CAD build for the part. Positions are in the model's coordinates, mm. Face numbers are marked on the shaded views. A direction names the side the tool comes from. Give positions to 0.01 mm unless a question says otherwise; leave off trailing zeros. Loops run counter-clockwise (first coordinate to the right, second up) from the corner with the lowest first, then second, coordinate; pieces in that order, holes last. Notation, with made-up numbers: (60, 83) - (82, 83) arc R34 ccw to (82, 115) - close; hole circle Ø5 at (-28.75, 88.25). An arc over 180 degrees is marked (long way). Return JSON: item names as keys, results as strings.
from build123d import *

# Parameters (mm, degrees)
SKETCH1_W           = 80
SKETCH1_H           = 160
BOSS_EXTRUDE1_DEPTH = 80
SHELL1_T            = -3
SKETCH2_W           = 40
SKETCH2_H           = 30
CUT_EXTRUDE1_DEPTH  = 70
SKETCH3_W           = 20
SKETCH3_H           = 15
CUT_EXTRUDE2_DEPTH  = 70
SKETCH4_W           = 70
SKETCH4_H           = 15
CUT_EXTRUDE3_DEPTH  = 70
SKETCH5_W           = 20
SKETCH5_H           = 10
SKETCH5_R           = 2
BOSS_EXTRUDE2_DEPTH = 3
SKETCH6_R           = 2
CUT_EXTRUDE4_DEPTH  = 3


with BuildPart() as part:
    # Sketch1 → Boss-Extrude1 (new body)
    with BuildSketch(Plane.XY):
        Rectangle(SKETCH1_W, SKETCH1_H)
    extrude(amount=BOSS_EXTRUDE1_DEPTH)

    # Shell1
    shell1_openings = [part.faces().sort_by_distance(p)[0] for p in [
        (0, 0, 0),
    ]]
    offset(amount=SHELL1_T, openings=shell1_openings, kind=Kind.INTERSECTION)

    # Sketch2 → Cut-Extrude1 (cut)
    with BuildSketch(Plane(origin=(0, 80, 0), x_dir=(1, 0, 0), z_dir=(0, 1, 0))):
        with Locations((0, -50)):
            Rectangle(SKETCH2_W, SKETCH2_H)
    extrude(amount=-CUT_EXTRUDE1_DEPTH, mode=Mode.SUBTRACT)

    # Sketch3 → Cut-Extrude2 (cut)
    with BuildSketch(Plane(origin=(0, 80, 0), x_dir=(1, 0, 0), z_dir=(0, 1, 0))):
        with Locations((0, -7.5)):
            Rectangle(SKETCH3_W, SKETCH3_H)
    extrude(amount=-CUT_EXTRUDE2_DEPTH, mode=Mode.SUBTRACT)

    # Sketch4 → Cut-Extrude3 (cut)
    with BuildSketch(Plane(origin=(0, -80, 0), x_dir=(-1, 0, 0), z_dir=(0, -1, 0))):
        with Locations((0, -7.5)):
            Rectangle(SKETCH4_W, SKETCH4_H)
    extrude(amount=-CUT_EXTRUDE3_DEPTH, mode=Mode.SUBTRACT)

    # Sketch5 → Boss-Extrude2 (add)
    # profile 1 of 2: a face of its own
    with BuildSketch(Plane(origin=(0, 0, 0), x_dir=(-1, 0, 0), z_dir=(0, 0, -1))):
        with Locations((50, 60)):
            Rectangle(SKETCH5_W, SKETCH5_H)
        with Locations((55, 60)):
            Circle(SKETCH5_R, mode=Mode.SUBTRACT)
    # profile 2 of 2: a face of its own
    with BuildSketch(Plane(origin=(0, 0, 0), x_dir=(-1, 0, 0), z_dir=(0, 0, -1))):
        with Locations((50, -70)):
            Rectangle(SKETCH5_W, SKETCH5_H)
        with Locations((55, -70)):
            Circle(SKETCH5_R, mode=Mode.SUBTRACT)
    boss_extrude2 = extrude(amount=-BOSS_EXTRUDE2_DEPTH)

    # Mirror1: Boss-Extrude2 across plane
    add(boss_extrude2.mirror(Plane(origin=(0, 0, 0), x_dir=(0, 0, 1), z_dir=(1, 0, 0))))

    # Sketch6 → Cut-Extrude4 (cut)
    with BuildSketch(Plane(origin=(0, 80, 0), x_dir=(1, 0, 0), z_dir=(0, 1, 0))):
        with Locations(Location((-27.5, -28, 0), (0, 0, 270))):
            Circle(SKETCH6_R)
        with Locations(Location((27.5, -28, 0), (0, 0, 270))):
            Circle(SKETCH6_R)
        with Locations(Location((27.5, -73, 0), (0, 0, 270))):
            Circle(SKETCH6_R)
        with Locations(Location((-27.5, -73, 0), (0, 0, 270))):
            Circle(SKETCH6_R)
    extrude(amount=-CUT_EXTRUDE4_DEPTH, mode=Mode.SUBTRACT)


solid = part.part
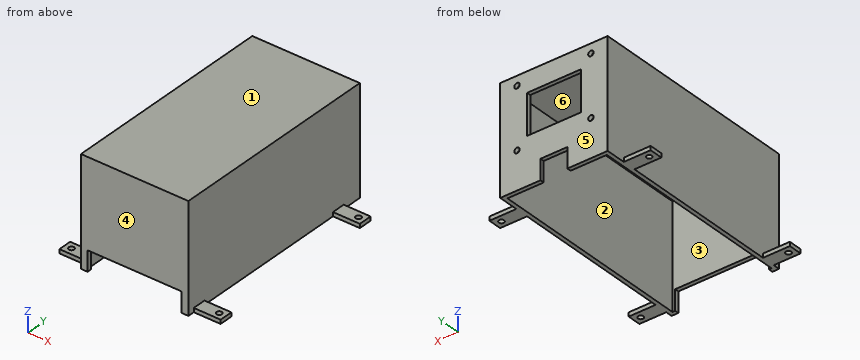
1. Cut at A-A, the plane z = 73. Write the cut outline in (x, y).
Values follow:
{"outline": "(-40, -80) - (40, -80) - (40, 80) - (29.5, 80) - (29.5, 77) - (37, 77) - (37, -77) - (-37, -77) - (-37, 77) - (-29.5, 77) - (-29.5, 80) - (-40, 80) - close; (-25.5, 77) - (25.5, 77) - (25.5, 80) - (-25.5, 80) - close"}
2. Pull direction Y, two halves, no side cores. Call the marked faces 3, 4, 5 and 6: +Y half, -Y half, draft (parallel to the pull), parting line (faces both ways), or undercut.
Values follow:
{"face 3": "undercut", "face 4": "-Y half", "face 5": "+Y half", "face 6": "undercut"}
3. Cut at B-B, the plane y = -70. Write the cut outline in (x, z).
Values follow:
{"outline": "(-60, 0) - (-57, 0) - (-57, 3) - (-60, 3) - close; (-53, 0) - (-37, 0) - (-37, 77) - (37, 77) - (37, 0) - (53, 0) - (53, 3) - (40, 3) - (40, 80) - (-40, 80) - (-40, 3) - (-53, 3) - close; (57, 0) - (60, 0) - (60, 3) - (57, 3) - close"}
4. Cut at D-D, the plane x = 42. Write the cut outline in (y, z).
Values follow:
{"outline": "(-75, 0) - (-65, 0) - (-65, 3) - (-75, 3) - close; (55, 0) - (65, 0) - (65, 3) - (55, 3) - close"}
5. Drill centre lines: probe 1 along X at (y, z) = (77.65, 28); probe 2 along Y at (x, z) = (-55, 1.2); probe 3 along X at (y, z) = (-19.5, 34.5). Where is each one in solid material? Low to high.
Values follow:
{"probe 1": "x = -40 to -29.5, -25.5 to 25.5, 29.5 to 40", "probe 2": "y = -75 to -72, -68 to -65, 55 to 58, 62 to 65", "probe 3": "x = -40 to -37, 37 to 40"}
6. Which spindle directions (+Z, -Z, +X, -X, +Y, -Y) get a long thin tool onto all of the face, cutting with end or side? Do the marked faces 1 and 2. Say none if no direction does.
Values follow:
{"face 1": "+Z, +X, -X, +Y, -Y", "face 2": "-Z"}
7. Cut at C-C, the plane x = 55. Write the cut outline in (y, z), plus the area to 3 significant figures.
Values follow:
{"outline": "(-75, 0) - (-72, 0) - (-72, 3) - (-75, 3) - close; (-68, 0) - (-65, 0) - (-65, 3) - (-68, 3) - close; (55, 0) - (58, 0) - (58, 3) - (55, 3) - close; (62, 0) - (65, 0) - (65, 3) - (62, 3) - close", "area": "36.0 mm²"}
8. Drop flat-ended pins along their axis: P1, Ø5, axis at x = 47, y = 58.5, coming from the +Z side; P2, Ø2.5, axis at x = -4, y = 78.5, coming from the -Z side; P3, Ø1, axis at x = 24.5, y = 31.5, coming from the -Z side. Give the stop position or say it passes through.
Values follow:
{"P1": "stops at z = 3", "P2": "stops at z = 15", "P3": "stops at z = 77"}
